Read the model definition and answer for the solid it produces. Units are mm, in the model's axes. A direction names the side the tool comes from. Give positions to 0.01 mm unless a question says otherwise; leave off trailing zeros. Order: outer loops, then holes, each group sorted by start corner. A loop starts at its lowest first (then second) coordinate and runs counter-clockwise, first axis right, second up. Notation, with made-up numbers: (-3, 84) - (45, 84) arc R38 cw to (45, 122) - close; hole circle Ø4 at (63, 28). An arc over 180 degrees is marked (long way). Write item = value, one per line.
```python
from build123d import *

# Parameters (mm, degrees)
SKETCH1_W           = 172
SKETCH1_H           = 119.2019
BOSS_EXTRUDE1_DEPTH = 8
CUT_EXTRUDE1_REACH  = 211.421
SKETCH2_R           = 6.5
SKETCH2_R_2         = 1.9
SKETCH2_R_3         = 2.1
SKETCH3_R           = 2.1
CUT_EXTRUDE2_DEPTH  = 15
CUT_EXTRUDE3_START  = -104.2019
SKETCH3_3_R         = 2.1
CUT_EXTRUDE3_DEPTH  = 15
CUT_EXTRUDE4_REACH  = 211.421
SKETCH4_R           = 1.55


with BuildPart() as part:
    # Sketch1 → Boss-Extrude1 (new body)
    with BuildSketch(Plane(origin=(0, 0, 0), x_dir=(-1, 0, 0), z_dir=(0, 1, 0))):
        with Locations((86, 59.60095)):
            Rectangle(SKETCH1_W, SKETCH1_H)
    extrude(amount=BOSS_EXTRUDE1_DEPTH)

    # Sketch2 → Cut-Extrude1 (cut, up to next)
    with BuildSketch(Plane.XZ, mode=Mode.PRIVATE) as cut_extrude1_sk1:
        with Locations(Location((-45.35, 68.7019, 0), (0, 0, 270))):
            Circle(SKETCH2_R)
    cut_extrude1_tool1 = extrude(cut_extrude1_sk1.sketch, amount=-CUT_EXTRUDE1_REACH, mode=Mode.PRIVATE) & part.part
    # Sketch2 → Cut-Extrude1 (cut, up to next)
    with BuildSketch(Plane.XZ, mode=Mode.PRIVATE) as cut_extrude1_sk2:
        with Locations(Location((-60.85, 75.7019, 0), (0, 0, 270))):
            Circle(SKETCH2_R_2)
    cut_extrude1_tool2 = extrude(cut_extrude1_sk2.sketch, amount=-CUT_EXTRUDE1_REACH, mode=Mode.PRIVATE) & part.part
    # Sketch2 → Cut-Extrude1 (cut, up to next)
    with BuildSketch(Plane.XZ, mode=Mode.PRIVATE) as cut_extrude1_sk3:
        with Locations(Location((-53.1, 89.125293759, 0), (0, 0, 270))):
            Circle(SKETCH2_R_2)
    cut_extrude1_tool3 = extrude(cut_extrude1_sk3.sketch, amount=-CUT_EXTRUDE1_REACH, mode=Mode.PRIVATE) & part.part
    # Sketch2 → Cut-Extrude1 (cut, up to next)
    with BuildSketch(Plane.XZ, mode=Mode.PRIVATE) as cut_extrude1_sk4:
        with Locations(Location((-37.6, 89.125293759, 0), (0, 0, 270))):
            Circle(SKETCH2_R_2)
    cut_extrude1_tool4 = extrude(cut_extrude1_sk4.sketch, amount=-CUT_EXTRUDE1_REACH, mode=Mode.PRIVATE) & part.part
    # Sketch2 → Cut-Extrude1 (cut, up to next)
    with BuildSketch(Plane.XZ, mode=Mode.PRIVATE) as cut_extrude1_sk5:
        with Locations(Location((-29.85, 75.7019, 0), (0, 0, 270))):
            Circle(SKETCH2_R_2)
    cut_extrude1_tool5 = extrude(cut_extrude1_sk5.sketch, amount=-CUT_EXTRUDE1_REACH, mode=Mode.PRIVATE) & part.part
    # Sketch2 → Cut-Extrude1 (cut, up to next)
    with BuildSketch(Plane.XZ, mode=Mode.PRIVATE) as cut_extrude1_sk6:
        with Locations(Location((-37.6, 62.278506241, 0), (0, 0, 270))):
            Circle(SKETCH2_R_2)
    cut_extrude1_tool6 = extrude(cut_extrude1_sk6.sketch, amount=-CUT_EXTRUDE1_REACH, mode=Mode.PRIVATE) & part.part
    # Sketch2 → Cut-Extrude1 (cut, up to next)
    with BuildSketch(Plane.XZ, mode=Mode.PRIVATE) as cut_extrude1_sk7:
        with Locations(Location((-53.1, 62.278506241, 0), (0, 0, 270))):
            Circle(SKETCH2_R_2)
    cut_extrude1_tool7 = extrude(cut_extrude1_sk7.sketch, amount=-CUT_EXTRUDE1_REACH, mode=Mode.PRIVATE) & part.part
    # Sketch2 → Cut-Extrude1 (cut, up to next)
    with BuildSketch(Plane.XZ, mode=Mode.PRIVATE) as cut_extrude1_sk8:
        with Locations(Location((-76.6, 68.7019, 0), (0, 0, 270))):
            Circle(SKETCH2_R_3)
    cut_extrude1_tool8 = extrude(cut_extrude1_sk8.sketch, amount=-CUT_EXTRUDE1_REACH, mode=Mode.PRIVATE) & part.part
    # Sketch2 → Cut-Extrude1 (cut, up to next)
    with BuildSketch(Plane.XZ, mode=Mode.PRIVATE) as cut_extrude1_sk9:
        with Locations(Location((-14.1, 68.7019, 0), (0, 0, 270))):
            Circle(SKETCH2_R_3)
    cut_extrude1_tool9 = extrude(cut_extrude1_sk9.sketch, amount=-CUT_EXTRUDE1_REACH, mode=Mode.PRIVATE) & part.part
    # Sketch2 → Cut-Extrude1 (cut, up to next)
    with BuildSketch(Plane.XZ, mode=Mode.PRIVATE) as cut_extrude1_sk10:
        with Locations(Location((-70.5, 54.2019, 0), (0, 0, 270))):
            Circle(SKETCH2_R_3)
    cut_extrude1_tool10 = extrude(cut_extrude1_sk10.sketch, amount=-CUT_EXTRUDE1_REACH, mode=Mode.PRIVATE) & part.part
    # Sketch2 → Cut-Extrude1 (cut, up to next)
    with BuildSketch(Plane.XZ, mode=Mode.PRIVATE) as cut_extrude1_sk11:
        with Locations(Location((-101.5, 54.2019, 0), (0, 0, 270))):
            Circle(SKETCH2_R_3)
    cut_extrude1_tool11 = extrude(cut_extrude1_sk11.sketch, amount=-CUT_EXTRUDE1_REACH, mode=Mode.PRIVATE) & part.part
    # Sketch2 → Cut-Extrude1 (cut, up to next)
    with BuildSketch(Plane.XZ, mode=Mode.PRIVATE) as cut_extrude1_sk12:
        with BuildLine():
            Line((-160.121320344, 89.110016908), (-138.908116908, 110.323220344))
            ThreePointArc((-138.908116908, 110.323220344), (-134.665476221, 110.323220344), (-134.665476221, 106.080579656))
            Line((-134.665476221, 106.080579656), (-155.878679656, 84.867376221))
            ThreePointArc((-155.878679656, 84.867376221), (-160.121320344, 84.867376221), (-160.121320344, 89.110016908))
        make_face()
    cut_extrude1_tool12 = extrude(cut_extrude1_sk12.sketch, amount=-CUT_EXTRUDE1_REACH, mode=Mode.PRIVATE) & part.part
    # Sketch2 → Cut-Extrude1 (cut, up to next)
    with BuildSketch(Plane.XZ, mode=Mode.PRIVATE) as cut_extrude1_sk13:
        with BuildLine():
            Line((-160.121320344, 74.967881284), (-124.765981284, 110.323220344))
            ThreePointArc((-124.765981284, 110.323220344), (-120.523340597, 110.323220344), (-120.523340597, 106.080579656))
            Line((-120.523340597, 106.080579656), (-155.878679656, 70.725240597))
            ThreePointArc((-155.878679656, 70.725240597), (-160.121320344, 70.725240597), (-160.121320344, 74.967881284))
        make_face()
    cut_extrude1_tool13 = extrude(cut_extrude1_sk13.sketch, amount=-CUT_EXTRUDE1_REACH, mode=Mode.PRIVATE) & part.part
    # Sketch2 → Cut-Extrude1 (cut, up to next)
    with BuildSketch(Plane.XZ, mode=Mode.PRIVATE) as cut_extrude1_sk14:
        with BuildLine():
            Line((-160.121320344, 60.825745661), (-110.623845661, 110.323220344))
            ThreePointArc((-110.623845661, 110.323220344), (-106.381204973, 110.323220344), (-106.381204973, 106.080579656))
            Line((-106.381204973, 106.080579656), (-155.878679656, 56.583104973))
            ThreePointArc((-155.878679656, 56.583104973), (-160.121320344, 56.583104973), (-160.121320344, 60.825745661))
        make_face()
    cut_extrude1_tool14 = extrude(cut_extrude1_sk14.sketch, amount=-CUT_EXTRUDE1_REACH, mode=Mode.PRIVATE) & part.part
    # Sketch2 → Cut-Extrude1 (cut, up to next)
    with BuildSketch(Plane.XZ, mode=Mode.PRIVATE) as cut_extrude1_sk15:
        with BuildLine():
            Line((-160.121320344, 46.683610037), (-96.481710037, 110.323220344))
            ThreePointArc((-96.481710037, 110.323220344), (-92.23906935, 110.323220344), (-92.23906935, 106.080579656))
            Line((-92.23906935, 106.080579656), (-155.878679656, 42.44096935))
            ThreePointArc((-155.878679656, 42.44096935), (-160.121320344, 42.44096935), (-160.121320344, 46.683610037))
        make_face()
    cut_extrude1_tool15 = extrude(cut_extrude1_sk15.sketch, amount=-CUT_EXTRUDE1_REACH, mode=Mode.PRIVATE) & part.part
    # Sketch2 → Cut-Extrude1 (cut, up to next)
    with BuildSketch(Plane.XZ, mode=Mode.PRIVATE) as cut_extrude1_sk16:
        with BuildLine():
            Line((-160.121320344, 103.252152532), (-153.050252532, 110.323220344))
            ThreePointArc((-153.050252532, 110.323220344), (-148.807611845, 110.323220344), (-148.807611845, 106.080579656))
            Line((-148.807611845, 106.080579656), (-155.878679656, 99.009511845))
            ThreePointArc((-155.878679656, 99.009511845), (-160.121320344, 99.009511845), (-160.121320344, 103.252152532))
        make_face()
    cut_extrude1_tool16 = extrude(cut_extrude1_sk16.sketch, amount=-CUT_EXTRUDE1_REACH, mode=Mode.PRIVATE) & part.part
    add(cut_extrude1_tool1.solids().sort_by_distance((-45.35, 0, 68.7019))[0], mode=Mode.SUBTRACT)
    add(cut_extrude1_tool2.solids().sort_by_distance((-60.85, 0, 75.7019))[0], mode=Mode.SUBTRACT)
    add(cut_extrude1_tool3.solids().sort_by_distance((-53.1, 0, 89.125294))[0], mode=Mode.SUBTRACT)
    add(cut_extrude1_tool4.solids().sort_by_distance((-37.6, 0, 89.125294))[0], mode=Mode.SUBTRACT)
    add(cut_extrude1_tool5.solids().sort_by_distance((-29.85, 0, 75.7019))[0], mode=Mode.SUBTRACT)
    add(cut_extrude1_tool6.solids().sort_by_distance((-37.6, 0, 62.278506))[0], mode=Mode.SUBTRACT)
    add(cut_extrude1_tool7.solids().sort_by_distance((-53.1, 0, 62.278506))[0], mode=Mode.SUBTRACT)
    add(cut_extrude1_tool8.solids().sort_by_distance((-76.6, 0, 68.7019))[0], mode=Mode.SUBTRACT)
    add(cut_extrude1_tool9.solids().sort_by_distance((-14.1, 0, 68.7019))[0], mode=Mode.SUBTRACT)
    add(cut_extrude1_tool10.solids().sort_by_distance((-70.5, 0, 54.2019))[0], mode=Mode.SUBTRACT)
    add(cut_extrude1_tool11.solids().sort_by_distance((-101.5, 0, 54.2019))[0], mode=Mode.SUBTRACT)
    add(cut_extrude1_tool12.solids().sort_by_distance((-147.393398, 0, 97.595298))[0], mode=Mode.SUBTRACT)
    add(cut_extrude1_tool13.solids().sort_by_distance((-140.32233, 0, 90.52423))[0], mode=Mode.SUBTRACT)
    add(cut_extrude1_tool14.solids().sort_by_distance((-133.251263, 0, 83.453163))[0], mode=Mode.SUBTRACT)
    add(cut_extrude1_tool15.solids().sort_by_distance((-126.180195, 0, 76.382095))[0], mode=Mode.SUBTRACT)
    add(cut_extrude1_tool16.solids().sort_by_distance((-154.464466, 0, 104.666366))[0], mode=Mode.SUBTRACT)

    # Sketch3 → Cut-Extrude2 (cut)
    with BuildSketch(Plane(origin=(0, 0, 0), x_dir=(1, 0, 0), z_dir=(0, 0, -1))):
        with Locations(Location((-5, -4, 0), (0, 0, 180))):
            Circle(SKETCH3_R)
        with Locations(Location((-167, -4, 0), (0, 0, 180))):
            Circle(SKETCH3_R)
        with Locations(Location((-86, -4, 0), (0, 0, 180))):
            Circle(SKETCH3_R)
    extrude(amount=-CUT_EXTRUDE2_DEPTH, mode=Mode.SUBTRACT)

    # Sketch3<3> → Cut-Extrude3 (cut)
    with BuildSketch(Plane(origin=(0, 0, 0), x_dir=(1, 0, 0), z_dir=(0, 0, -1)).offset(CUT_EXTRUDE3_START)):
        with Locations(Location((-5, -4, 0), (0, 0, 180))):
            Circle(SKETCH3_3_R)
        with Locations(Location((-167, -4, 0), (0, 0, 180))):
            Circle(SKETCH3_3_R)
        with Locations(Location((-86, -4, 0), (0, 0, 180))):
            Circle(SKETCH3_3_R)
    extrude(amount=-CUT_EXTRUDE3_DEPTH, mode=Mode.SUBTRACT)

    # Sketch4 → Cut-Extrude4 (cut, up to next)
    with BuildSketch(Plane.XZ, mode=Mode.PRIVATE) as cut_extrude4_sk1:
        with Locations(Location((-168, 84.60095, 0), (0, 0, 270))):
            Circle(SKETCH4_R)
    cut_extrude4_tool1 = extrude(cut_extrude4_sk1.sketch, amount=-CUT_EXTRUDE4_REACH, mode=Mode.PRIVATE) & part.part
    # Sketch4 → Cut-Extrude4 (cut, up to next)
    with BuildSketch(Plane.XZ, mode=Mode.PRIVATE) as cut_extrude4_sk2:
        with Locations(Location((-168, 34.60095, 0), (0, 0, 270))):
            Circle(SKETCH4_R)
    cut_extrude4_tool2 = extrude(cut_extrude4_sk2.sketch, amount=-CUT_EXTRUDE4_REACH, mode=Mode.PRIVATE) & part.part
    # Sketch4 → Cut-Extrude4 (cut, up to next)
    with BuildSketch(Plane.XZ, mode=Mode.PRIVATE) as cut_extrude4_sk3:
        with Locations(Location((-4, 34.60095, 0), (0, 0, 270))):
            Circle(SKETCH4_R)
    cut_extrude4_tool3 = extrude(cut_extrude4_sk3.sketch, amount=-CUT_EXTRUDE4_REACH, mode=Mode.PRIVATE) & part.part
    # Sketch4 → Cut-Extrude4 (cut, up to next)
    with BuildSketch(Plane.XZ, mode=Mode.PRIVATE) as cut_extrude4_sk4:
        with Locations(Location((-4, 84.60095, 0), (0, 0, 270))):
            Circle(SKETCH4_R)
    cut_extrude4_tool4 = extrude(cut_extrude4_sk4.sketch, amount=-CUT_EXTRUDE4_REACH, mode=Mode.PRIVATE) & part.part
    add(cut_extrude4_tool1.solids().sort_by_distance((-168, 0, 84.60095))[0], mode=Mode.SUBTRACT)
    add(cut_extrude4_tool2.solids().sort_by_distance((-168, 0, 34.60095))[0], mode=Mode.SUBTRACT)
    add(cut_extrude4_tool3.solids().sort_by_distance((-4, 0, 34.60095))[0], mode=Mode.SUBTRACT)
    add(cut_extrude4_tool4.solids().sort_by_distance((-4, 0, 84.60095))[0], mode=Mode.SUBTRACT)


solid = part.part
```
1. Determine the mould class of faces 1 (the face through (-39.286, 3.944, 61.402)), 2 (the face through (-85, 0, 60)), 3 (the face through (-4.54, 1.95, 7.4)) for opening direction Y: +Y half, -Y half, draft (parallel to the pull), parting line (faces both ways), or undercut.
Recorded:
face_1 = draft
face_2 = -Y half
face_3 = undercut
2. Straight lines are drawn through the part: L1, parallel to Z at x = -38, y = 4.75; L2, parallel to X at y = 1.75, z = 56; L3, parallel to X at y = 5.75, z = 57. For each, find the intervals that lie inside material, in ascending order. Write a range as [from, to].
Recorded:
L1 = [0, 60.42], [64.14, 87.27], [90.98, 119.2]
L2 = [-172, -159.3], [-156.7, -150.8], [-142.32, -102.58], [-100.42, -71.58], [-69.42, 0]
L3 = [-172, -160.47], [-155.46, -149.8], [-141.32, 0]
3. Flat-ended cylindrical pins translate along their axes: pin 1 (1.3 mm diameter, centred on x = -6, y = 3, fed in from +Z); pin 2 (1.5 mm diameter, centred on y = 4, z = 64, fed in from +X). Find the tip coordinate at first contact, or state that the pin passes through.
Recorded:
pin_1 = 104.2
pin_2 = 0
4. Section B-B (x = -117.5) is taken. Determine the outline of the cut face in (y, z).
Recorded:
outline = (0, 0) - (8, 0) - (8, 80.82) - (0, 80.82) - close; (0, 89.3) - (8, 89.3) - (8, 94.96) - (0, 94.96) - close; (0, 103.45) - (8, 103.45) - (8, 119.2) - (0, 119.2) - close
5. Section D-D (x = -45.35) is taken. Determine the outline of the cut face in (y, z).
Recorded:
outline = (0, 0) - (8, 0) - (8, 62.2) - (0, 62.2) - close; (0, 75.2) - (8, 75.2) - (8, 119.2) - (0, 119.2) - close
6. Section A-A (x = -14.1) is taken. Determine the outline of the cut face in (y, z).
Recorded:
outline = (0, 0) - (8, 0) - (8, 66.6) - (0, 66.6) - close; (0, 70.8) - (8, 70.8) - (8, 119.2) - (0, 119.2) - close
7. Section C-C (x = -86) is taken. Determine the outline of the cut face in (y, z).
Recorded:
outline = (0, 0) - (1.9, 0) - (1.9, 15) - (6.1, 15) - (6.1, 0) - (8, 0) - (8, 119.2) - (6.1, 119.2) - (6.1, 104.2) - (1.9, 104.2) - (1.9, 119.2) - (0, 119.2) - close
8. For faces 4 (the face through (-135.719, 3.944, 85.228)), 5 (the face through (-168.94, 3.2, 111.6)), determine the directions among +Z, -Z, +X, -X, +Y, -Y from which every point of the face is accessible in a straight line to the end or side of a thin tool.
Recorded:
face_4 = +Y, -Y
face_5 = +Z
